```python
from build123d import *

# Parameters (mm, degrees)
F2_W     = 5
F2_H     = 4
F3_DEPTH = 212
F4_R     = 2.49999


# Not quite as in the source:
# - a fillet or chamfer is up to 0.001 mm smaller than in the source, because OpenCascade refuses the exact size
# - a feature names something its author has since deleted; it is built from what else it names


with BuildPart() as f1:
    # F0 (on Front) → F1 (revolve)
    with BuildSketch(Plane.XZ):
        Polygon((0, 12), (0, 16), (-230, 16), (-230, 11.9125), (-149.8207171315, 9.9), (-25, 9.9), (-25, 12), align=None)
    revolve(axis=Axis((-16.2521931838, 0, 0), (-1, 0, 0)))

    # F2 (on Right) → F3 (cut)
    with BuildSketch(Plane.YZ):
        with Locations((0, 14.5)):
            Rectangle(F2_W, F2_H)
    extrude(amount=-F3_DEPTH, mode=Mode.SUBTRACT)

    # F4 (radius 2.5 in the source; OpenCascade refuses exactly that, so slightly less here)
    f4_edges = [f1.edges().sort_by_distance(p)[0] for p in [
        (-212, 2.5, 14.15174),
        (-212, -2.5, 14.15174),
    ]]
    fillet(f4_edges, radius=F4_R)


solid = f1.part
```
Geometry check sheet. Reference: the model listing, model coordinates, mm. A direction names the side the tool comes from. Round coordinates to 2 decimals unless told otherwise and drop trailing zeros. Loops run counter-clockwise (first coordinate to the right, second up) from the corner with the lowest first, then second, coordinate; pieces in that order, holes last. Notation, with made-up numbers: M -39,65.5 L -35,65.5 A31 ccw -35,101.5 Z; hole C 25.25,-30.5 d4. An arc over 180 degrees is marked long. Return JSON: item names as keys, results as strings. Group by question number.
(1) Mould release check, pull along Y, two halves, no side actions. Record for faces 4 (the face through (-189.349, -10.633, -2.361)), 5 (the face through (-116.61, -15.62, -3.47)), 6 (the face through (-230, 12, -2)), 7 (the face through (-25, 10, -2)): pulls with the +Y half, pulls with the -Y half, needs draft (parallel to the pull), parting line crosses it, or undercut.
(2) Scan lines: line 1 along Y through (x, z) = (-10, 0); line 2 along Y through (x, z) = (-121, 0); line 3 along Z through (x, y) = (-13, 1). Record each from-to range of solid material in increasing order. Write a range as [from, to].
(3) Go/stop test with flat-tipped pins: pin 1 (8 mm diameter, centred on x = -67, y = -10.5, fed in from -Z); pin 2 (2.5 mm diameter, centred on x = -68, y = 0.5, fed in from +Z); pin 3 (5 mm diameter, centred on x = -186, y = -6, fed in from -Z). Record where each tip stops, or that it passes through.
(4) Set-up check for faces 1 (the face through (-12.32, 0.53, -11.99)), 2 (the face through (-105, 0, 12.5)), 3 (the face through (-86.537, 2.974, 9.443)): record each of +Z, -Z, +X, -X, +Y, -Y from which the full face is reachable in a straight line by a thin tool's end or side.
(5) Section check A-A, the plane z = 0. Enter the section's corners in (x, y).
(6) Section check C-C, the plane x = -200. Enter the section's corners in (y, z).
(7) Section check B-B, the plane x = -144. Enter the section's corners in (y, z).
Data:
{
 "1": {"face 4": "undercut", "face 5": "parting line crosses it", "face 6": "needs draft", "face 7": "undercut"},
 "2": {"line 1": "[-16, -12], [12, 16]", "line 2": "[-16, -9.9], [9.9, 16]", "line 3": "[-15.97, -11.96], [11.96, 12.5]"},
 "3": {"pin 1": "z = -14.62", "pin 2": "z = 12.5", "pin 3": "z = -15.61"},
 "4": {"face 1": "+X", "face 2": "+Z, +X", "face 3": "+X, -X"},
 "5": {"outline": "M -230,-16 L 0,-16 L 0,-12 L -25,-12 L -25,-9.9 L -149.82,-9.9 L -230,-11.91 Z; M -230,11.91 L -149.82,9.9 L -25,9.9 L -25,12 L 0,12 L 0,16 L -230,16 Z"},
 "6": {"outline": "M -2.5,12.5 L -2.5,15.8 A16 ccw long 2.5,15.8 L 2.5,12.5 Z; hole C 0,0 d22.32"},
 "7": {"outline": "M -2.5,12.5 L -2.5,15.8 A16 ccw long 2.5,15.8 L 2.5,12.5 Z; hole C 0,0 d19.8"}
}
